For this review, take the finished solid that the model builds, in its own axes (mm). A direction names the side the tool comes from. Give positions to 0.01 mm unless a question says otherwise; leave off trailing zeros. Loops run counter-clockwise (first coordinate to the right, second up) from the corner with the lowest first, then second, coordinate; pieces in that order, holes last.
```python
from build123d import *

# Parameters (mm, degrees)
F0_R           = 10
F1_DEPTH       = 80
F3_DEPTH       = 10
F6_R           = 14
F7_DEPTH       = 10
F9_R           = 14
F10_DEPTH      = 10
F12_R          = 14
F13_DEPTH      = 10
F15_R          = 14
F16_DEPTH      = 10
F17_R          = 20
F18_DEPTH      = 20
F22_DEPTH      = 25
F22_DEPTH_BACK = 25
F23_R          = 16
F24_DEPTH      = 25
F24_DEPTH_BACK = 25


with BuildPart() as f1:
    # F0 (on Top) → F1 (new body)
    with BuildSketch(Plane.XY):
        Circle(F0_R)
    extrude(amount=F1_DEPTH)

    # F2 (on Top) → F3 (join)
    with BuildSketch(Plane.XY):
        Polygon((14, 0), (5.9740389772, 12.6613924313), (-0.0259610228, 12.6613924313), (-5.9740389772, 12.6613924313), (-14, 0), (-5.9740389772, -12.6613924313), (0.0259610228, -12.6613924313), (5.9740389772, -12.6613924313), align=None)
    extrude(amount=F3_DEPTH)

    # F6 (on offset) → F7 (join)
    with BuildSketch(Plane.XY.offset(15)):
        Circle(F6_R)
    extrude(amount=F7_DEPTH)

    # F9 (on offset) → F10 (join)
    with BuildSketch(Plane.XY.offset(30)):
        Circle(F9_R)
    extrude(amount=F10_DEPTH)

    # F12 (on offset) → F13 (join)
    with BuildSketch(Plane.XY.offset(45)):
        Circle(F12_R)
    extrude(amount=F13_DEPTH)

    # F15 (on offset) → F16 (join)
    with BuildSketch(Plane.XY.offset(60)):
        Circle(F15_R)
    extrude(amount=F16_DEPTH)

    # F17 (on face) → F18 (join)
    with BuildSketch(Plane.XY.offset(70)):
        Circle(F17_R)
    extrude(amount=F18_DEPTH)

    # F19 (on face) → F20 (revolve, cut)
    with BuildSketch(Plane.XY.offset(90)):
        with BuildLine():
            Line((0, -13.8652793043), (0, 13.8652793043))
            ThreePointArc((0, 13.8652793043), (-13.8652793043, 0), (0, -13.8652793043))
        make_face()
    revolve(axis=Axis((0, 0, 90), (0, -1, 0)), mode=Mode.SUBTRACT)

    # F21 (on Front) → F22 (cut, two sides)
    with BuildSketch(Plane.XZ) as f22_sk:
        with BuildLine():
            Line((20.291691646, 89.9962559342), (20.291691646, 107.0001030122))
            ThreePointArc((20.291691646, 107.0001030122), (3.287844568, 89.9962559342), (20.291691646, 72.9924088562))
            Line((20.291691646, 72.9924088562), (20.291691646, 89.9962559342))
        make_face()
    extrude(amount=F22_DEPTH, mode=Mode.SUBTRACT)
    extrude(f22_sk.sketch, amount=-F22_DEPTH_BACK, mode=Mode.SUBTRACT)

    # F23 (on Front) → F24 (cut, two sides)
    with BuildSketch(Plane.XZ) as f24_sk:
        with Locations((-20.4308144748, 90.1330336928)):
            Circle(F23_R)
    extrude(amount=-F24_DEPTH, mode=Mode.SUBTRACT)
    extrude(f24_sk.sketch, amount=F24_DEPTH_BACK, mode=Mode.SUBTRACT)


solid = f1.part
```
Q1. Consider section D-D on z = 56.5. Give the boundary of the cut face in (x, y), plus the area to 3 significant figures.
Answers:
outline: circle Ø20 at (0, 0)
area: 314 mm2
Q2. Machinability: for faces 1 (the flat face through (9.93, -6.42, 4.93)), 2 (the flat face through (0, -12.661, 5)), 3 (the flat face through (10.043, 6.242, 4.93)), 4 (the flat face through (-3, 10, 60)), 5 (the flat face through (-14, -4, 70)), which of the approach directions +Z, -Z, +X, -X, +Y, -Y give a long, thin tool a straight path to every point of the face, cutting with its end or side? Answer none if there is none.
Answers:
face 1: -Z, +X, -Y
face 2: -Z, +X, -X, -Y
face 3: -Z, +X, +Y
face 4: none
face 5: -Z
Q3. Consider section A-A on y = 11. Give the boundary of the cut face in (x, z).
Answers:
outline: (-16.7, 70) - (-8.66, 70) - (-8.66, 60) - (8.66, 60) - (8.66, 70) - (16.7, 70) - (16.7, 73.38) arc R17 cw to (4.78, 83.04) arc R8.44 cw to (-5.73, 83.81) arc R16 cw to (-16.7, 74.57) - close; (-8.66, 15) - (8.66, 15) - (8.66, 25) - (-8.66, 25) - close; (-8.66, 30) - (8.66, 30) - (8.66, 40) - (-8.66, 40) - close; (-8.66, 45) - (8.66, 45) - (8.66, 55) - (-8.66, 55) - close; (-7.03, 0) - (7.03, 0) - (7.03, 10) - (-7.03, 10) - close
Q4. For pin 1 Ø10 at (y, z) = (12.5, 56.5) entering from -X; pin 2 Ø1 at (x, z) = (-5, 75.5) entering from -Y; pin 3 Ø2 at (x, z) = (8.5, 17.5) entering from +Y, all flat-tipped, find the tip position at first contact; note any pin that passes through.
Answers:
pin 1: stops at x = -11.67
pin 2: stops at y = -19.49
pin 3: stops at y = 11.82
Q5. Mouldability with a two-part tool opening along Z and no side actions: class faces 6 (the cylindrical face through (12.932, -5.362, 49.93)), 7 (the cylindrical face through (-2.17, -9.76, 12.46)), 8 (the cylindrical face through (-9.133, 0.273, 78.803)) as +Z half, -Z half, draft (parallel to the pull), parting line (faces both ways), or undercut.
Answers:
face 6: draft
face 7: undercut
face 8: +Z half
Q6. Consider section B-B on z = 7. Give the boundary of the cut face in (x, y), plus the area to 3 significant figures.
Answers:
outline: (-14, 0) - (-5.97, -12.66) - (5.97, -12.66) - (14, 0) - (5.97, 12.66) - (-5.97, 12.66) - close
area: 506 mm2
Q7. Consider section C-C on x = -15. Give the boundary of the cut face in (y, z).
Answers:
outline: (-13.23, 70) - (13.23, 70) - (13.23, 75.08) - (-13.23, 75.08) - close
Q8. For probe 1 along Z at (x, y) = (-8.5, 10); probe 2 along Z at (x, y) = (-10.5, 6); probe 3 along Y at (x, z) = (0.5, 66.5), list the stretches that pass through material, from the lowest coordinate up.
Answers:
probe 1: z = 15 to 25, 30 to 40, 45 to 55, 60 to 79.47
probe 2: z = 15 to 25, 30 to 40, 45 to 55, 60 to 77.59
probe 3: y = -13.99 to 13.99
